Job drawing, mm, ordinate dimensions from the low corner. One solid piece. A direction names the side the tool comes from. Coordinates: 2 decimals unless noted, no trailing zeros. Order: outer loops, then holes, each group sorted by start corner. A loop starts at its lowest first (then second) coordinate and runs counter-clockwise, first axis right, second up. Notation, with made-up numbers: (-22.5, -37.75) - (-5.5, -37.75) arc R4 ccw to (-5.5, -32.75) - close; hole circle Ø5 at (79.5, -34). An arc over 180 degrees is marked (long way). Return JSON: item names as keys, results as strings.
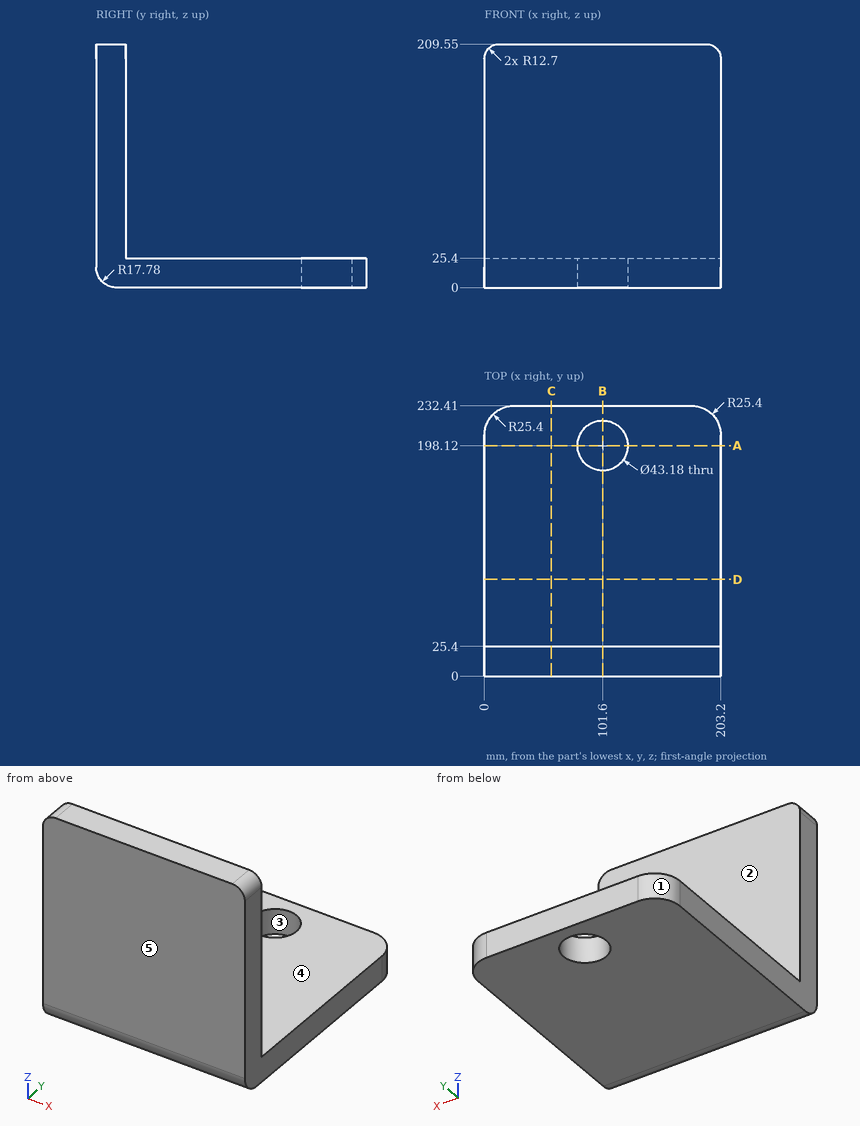
1. Cut at D-D on y = 83. Give the cut face in (x, z).
Check values:
{"outline": "(0, 0) - (203.2, 0) - (203.2, 25.4) - (0, 25.4) - close"}
2. Cut at A-A on y = 198.12. Give the cut face in (x, z).
Check values:
{"outline": "(0, 0) - (80.01, 0) - (80.01, 25.4) - (0, 25.4) - close; (123.19, 0) - (203.2, 0) - (203.2, 25.4) - (123.19, 25.4) - close"}
3. Tool access for the marked faces 4 and 5: list every direction of +Z, -Z, +X, -X, +Y, -Y with a clear straight run to the whole face (end or side of a thin tool).
Check values:
{"face 4": "+Z, +X, -X, +Y", "face 5": "+Z, -Z, +X, -X, -Y"}
4. Mould opens along X. For the marked faces 1, 2 and 3 say: pulls with the +X half, pulls with the -X half, needs draft (parallel to the pull), parting line crosses it, or undercut.
Check values:
{"face 1": "pulls with the -X half", "face 2": "needs draft", "face 3": "undercut"}
5. Probe L1, parallel to Z at x = 167.5, y = 201.5; L2, parallel to Y at x = 101, z = 17. List the from-to ranges inside material, lowest first.
Check values:
{"L1": "0 to 25.4", "L2": "0.02 to 176.54, 219.7 to 232.41"}
6. Drop flat-ended pins along their axis: pin 1 (6 mm diameter, centred on x = 41.5, y = 65.5, fed in from +Z); pin 2 (3 mm diameter, centred on x = 174.5, z = 44, fed in from +Y). Give the stop position or say it passes through.
Check values:
{"pin 1": "z = 25.4", "pin 2": "y = 25.4"}
7. Cut at B-B on x = 101.6. Give the cut face in (y, z).
Check values:
{"outline": "(0, 17.78) arc R17.78 ccw to (17.78, 0) - (176.53, 0) - (176.53, 25.4) - (25.4, 25.4) - (25.4, 209.55) - (0, 209.55) - close; (219.71, 0) - (232.41, 0) - (232.41, 25.4) - (219.71, 25.4) - close"}
8. Cut at C-C on x = 57.5. Give the cut face in (y, z).
Check values:
{"outline": "(0, 17.78) arc R17.78 ccw to (17.78, 0) - (232.41, 0) - (232.41, 25.4) - (25.4, 25.4) - (25.4, 209.55) - (0, 209.55) - close"}
